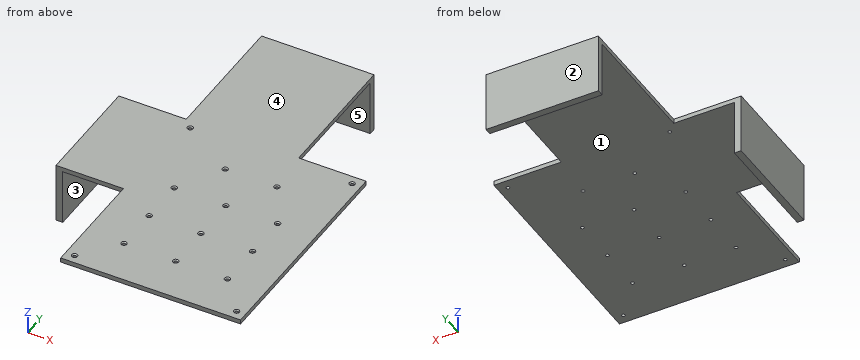
```python
from build123d import *

# Parameters (mm, degrees)
F0_W     = 80
F0_H     = 100
F0_R     = 0.75
F1_DEPTH = 2
F3_W     = 50
F3_H     = 2
F4_DEPTH = 60
F2_W     = 50
F2_H     = 2
F5_DEPTH = 30
F6_W     = 3
F6_H     = 50
F6_W_2   = 50
F6_H_2   = 3
F7_DEPTH = 25
F8_SIZE  = 0.5


with BuildPart() as f1:
    # F0 (on Top) → F1 (new body)
    with BuildSketch(Plane.XY):
        with Locations((-20.396638, -30.557484)):
            Rectangle(F0_W, F0_H)
        with Locations((-56.396638, -76.557484)):
            Circle(F0_R, mode=Mode.SUBTRACT)
        with Locations((-43.396638, -60.557484)):
            Circle(F0_R, mode=Mode.SUBTRACT)
        with Locations((-43.396638, -40.557484)):
            Circle(F0_R, mode=Mode.SUBTRACT)
        with Locations((-20.396638, -60.557484)):
            Circle(F0_R, mode=Mode.SUBTRACT)
        with Locations((15.603362, -76.557484)):
            Circle(F0_R, mode=Mode.SUBTRACT)
        with Locations((2.603362, -60.557484)):
            Circle(F0_R, mode=Mode.SUBTRACT)
        with Locations((-20.396638, -40.557484)):
            Circle(F0_R, mode=Mode.SUBTRACT)
        with Locations((2.603362, -40.557484)):
            Circle(F0_R, mode=Mode.SUBTRACT)
        with Locations((-43.396638, -20.557484)):
            Circle(F0_R, mode=Mode.SUBTRACT)
        with Locations((-56.396638, 15.442516)):
            Circle(F0_R, mode=Mode.SUBTRACT)
        with Locations((-31.896638, -0.557484)):
            Circle(F0_R, mode=Mode.SUBTRACT)
        with Locations((-20.396638, -20.557484)):
            Circle(F0_R, mode=Mode.SUBTRACT)
        with Locations((2.603362, -20.557484)):
            Circle(F0_R, mode=Mode.SUBTRACT)
        with Locations((-8.896638, -0.557484)):
            Circle(F0_R, mode=Mode.SUBTRACT)
        with Locations((15.603362, 15.442516)):
            Circle(F0_R, mode=Mode.SUBTRACT)
    extrude(amount=F1_DEPTH)

    # F3 (on face) → F4 (join)
    with BuildSketch(Plane(origin=(0, 19.442516, 0), x_dir=(-1, 0, 0), z_dir=(0, 1, 0))):
        with Locations((35.396638, 1)):
            Rectangle(F3_W, F3_H)
    extrude(amount=F4_DEPTH)

    # F2 (on face) → F5 (join)
    with BuildSketch(Plane(origin=(-60.396638, 0, 0), x_dir=(0, -1, 0), z_dir=(-1, 0, 0))):
        with Locations((5.557484, 1)):
            Rectangle(F2_W, F2_H)
    extrude(amount=F5_DEPTH)

    # F6 (on face) → F7 (join)
    with BuildSketch(Plane(origin=(0, 0, 0), x_dir=(1, 0, 0), z_dir=(0, 0, -1))):
        with Locations((-88.896638, 5.557484)):
            Rectangle(F6_W, F6_H)
        with Locations((-35.396638, -77.942516)):
            Rectangle(F6_W_2, F6_H_2)
    extrude(amount=F7_DEPTH)

    # F8
    f8_edges = [f1.edges().sort_by_distance(p)[0] for p in [
        (-57.146638, -76.557484, 2),
        (-44.146638, -60.557484, 2),
        (-44.146638, -40.557484, 2),
        (-44.146638, -20.557484, 2),
        (-32.646638, -0.557484, 2),
        (-21.146638, -20.557484, 2),
        (-21.146638, -40.557484, 2),
        (-21.146638, -60.557484, 2),
        (14.853362, -76.557484, 2),
        (1.853362, -60.557484, 2),
        (1.853362, -40.557484, 2),
        (1.853362, -20.557484, 2),
        (-9.646638, -0.557484, 2),
        (14.853362, 15.442516, 2),
        (-57.146638, 15.442516, 2),
    ]]
    chamfer(f8_edges, length=F8_SIZE)


solid = f1.part
```
Geometry check sheet. Reference: the model listing, model coordinates, mm. Face numbers are marked on the shaded views. A direction names the side the tool comes from. Coordinates: 2 decimals unless noted, no trailing zeros. Order: outer loops, then holes, each group sorted by start corner. A loop starts at its lowest first (then second) coordinate and runs counter-clockwise, first axis right, second up. Notation, with made-up numbers: (59, -34) - (89, -34) arc R29 cw to (89, 4) - close; hole circle Ø11 at (49.25, 21). An arc over 180 degrees is marked (long way). Answer as a JSON object with one key per item and string values. Group by question number.
Item 1: Sectioned sample at B-B, the plane x = -29. Record the cut outline in (y, z).
Item 2: Sectioned sample at C-C, the plane y = -36. Record the cut outline in (x, z), and give its area (3 significant figures).
Item 3: Depth check by flat-ended pin: pin 1 Ø2 at (x, y) = (-56.4, -76.56) entering from +Z; pin 2 Ø1.7 at (x, y) = (-8.9, -0.56) entering from -Z; pin 3 Ø1 at (x, z) = (-24, -13.5) entering from -Y. Enter the tip coordinate at first touch or a pass-through.
Item 4: Tool access check on the marked faces 1, 2, 3, 4 and 5. Record the directions out of +Z, -Z, +X, -X, +Y, -Y that give a thin tool (end or side, any length) a straight path to the whole face; none if there is none.
Item 5: Scan lines: probe 1 along X at (y, z) = (-19.5, -23); probe 2 along Z at (x, y) = (13, -28.5); probe 3 along Y at (x, z) = (-26.5, -13.25). Record each from-to range of solid material in increasing order.
Item 6: Sectioned sample at D-D, the plane x = -83.5. Record the cut outline in (y, z).
Item 7: Sectioned sample at A-A, the plane z = -14. Record the cut outline in (x, y), and give its area (3 significant figures).
Resolved:
{
 "1": {"outline": "(-80.56, 0) - (76.44, 0) - (76.44, -25) - (79.44, -25) - (79.44, 2) - (-80.56, 2) - close"},
 "2": {"outline": "(-60.4, 0) - (19.6, 0) - (19.6, 2) - (-60.4, 2) - close", "area": "160 mm^2"},
 "3": {"pin 1": "z = 1.75", "pin 2": "z = 0", "pin 3": "y = 76.44"},
 "4": {"face 1": "-Z, +X, -Y", "face 2": "+Z, -Z, +X, -X, +Y", "face 3": "-Z, +X, +Y, -Y", "face 4": "+Z, +X, -X, +Y, -Y", "face 5": "-Z, +X, -X, -Y"},
 "5": {"probe 1": "-90.4 to -87.4", "probe 2": "0 to 2", "probe 3": "76.44 to 79.44"},
 "6": {"outline": "(-30.56, 0) - (19.44, 0) - (19.44, 2) - (-30.56, 2) - close"},
 "7": {"outline": "(-90.4, -30.56) - (-87.4, -30.56) - (-87.4, 19.44) - (-90.4, 19.44) - close; (-60.4, 76.44) - (-10.4, 76.44) - (-10.4, 79.44) - (-60.4, 79.44) - close", "area": "300 mm^2"}
}
